Read the model definition and answer for the solid it produces. Units are mm, in the model's axes. A direction names the side the tool comes from. Coordinates: 2 decimals unless noted, no trailing zeros. Loops run counter-clockwise (first coordinate to the right, second up) from the corner with the lowest first, then second, coordinate; pieces in that order, holes last. Notation, with made-up numbers: M 59,69.25 L 72,69.25 A21 cw 72,76.25 Z; hole C -11.75,55.25 d10. An arc over 180 degrees is marked long. Put each result on its own line as item: value.
from build123d import *

# Parameters (mm, degrees)
F0_W     = 76.2
F0_H     = 38.1
F1_DEPTH = 2.032
F2_R     = 3.81
F3_DEPTH = 25.4
F2_W     = 71.628
F2_H     = 33.528
F2_W_2   = 67.564
F2_H_2   = 29.464
F4_DEPTH = 2.54
F5_R     = 5.08
F7_DEPTH = 25.4
F8_DEPTH = 25.4


with BuildPart() as f1:
    # F0 (on Top) → F1 (new body)
    with BuildSketch(Plane.XY):
        Rectangle(F0_W, F0_H)
    extrude(amount=F1_DEPTH)

    # F2 (on face) → F3 (cut)
    with BuildSketch(Plane.XY.offset(2.032)):
        Circle(F2_R)
    extrude(amount=-F3_DEPTH, mode=Mode.SUBTRACT)

    # F2 (on face) → F4 (join)
    with BuildSketch(Plane.XY.offset(2.032)):
        Rectangle(F2_W, F2_H)
        Rectangle(F2_W_2, F2_H_2, mode=Mode.SUBTRACT)
    extrude(amount=F4_DEPTH)

    # F5
    f5_edges = [f1.edges().sort_by_distance(p)[0] for p in [
        (-33.782, 14.732, 3.302),
        (-33.782, -14.732, 3.302),
        (33.782, -14.732, 3.302),
        (33.782, 14.732, 3.302),
        (-35.814, -16.764, 3.302),
        (-38.1, -19.05, 1.016),
        (38.1, -19.05, 1.016),
        (35.814, -16.764, 3.302),
        (38.1, 19.05, 1.016),
        (35.814, 16.764, 3.302),
        (-35.814, 16.764, 3.302),
        (-38.1, 19.05, 1.016),
    ]]
    fillet(f5_edges, radius=F5_R)

    # F6 (on face) → F7 (cut)
    with BuildSketch(Plane.XY.offset(2.032)):
        with BuildLine():
            ThreePointArc((22.9948570038, 2.5340882153), (21.082, 3.175), (19.1691429962, 2.5340882153))
            ThreePointArc((19.1691429962, 2.5340882153), (21.082, 2.1601883081), (22.9948570038, 2.5340882153))
        make_face()
        with BuildLine():
            ThreePointArc((19.1691429962, 2.5340882153), (18.2399984177, 1.4155041527), (17.907, 0))
            ThreePointArc((17.907, 0), (21.082, -3.175), (24.257, 0))
            ThreePointArc((24.257, 0), (23.9240015823, 1.4155041527), (22.9948570038, 2.5340882153))
            ThreePointArc((22.9948570038, 2.5340882153), (21.082, 2.1601883081), (19.1691429962, 2.5340882153))
        make_face()
        with BuildLine():
            ThreePointArc((17.907, 3.2746145791), (18.511267216, 2.8586665458), (19.1691429962, 2.5340882153))
            ThreePointArc((19.1691429962, 2.5340882153), (21.082, 3.175), (22.9948570038, 2.5340882153))
            ThreePointArc((22.9948570038, 2.5340882153), (23.652732784, 2.8586665458), (24.257, 3.2746145791))
            ThreePointArc((24.257, 3.2746145791), (25.6610501198, 5.0404837824), (26.162, 7.2401883081))
            ThreePointArc((26.162, 7.2401883081), (18.8822954744, 11.8192384279), (17.907, 3.2746145791))
        make_face()
        with BuildLine():
            Line((17.907, 3.2746145791), (17.907, 0))
            ThreePointArc((17.907, 0), (18.2399984177, 1.4155041527), (19.1691429962, 2.5340882153))
            ThreePointArc((19.1691429962, 2.5340882153), (18.511267216, 2.8586665458), (17.907, 3.2746145791))
        make_face()
        with BuildLine():
            ThreePointArc((22.9948570038, 2.5340882153), (23.9240015823, 1.4155041527), (24.257, 0))
            Line((24.257, 0), (24.257, 3.2746145791))
            ThreePointArc((24.257, 3.2746145791), (23.652732784, 2.8586665458), (22.9948570038, 2.5340882153))
        make_face()
    extrude(amount=-F7_DEPTH, mode=Mode.SUBTRACT)

    # F6 (on face) → F8 (cut)
    with BuildSketch(Plane.XY.offset(2.032)):
        with BuildLine():
            ThreePointArc((-24.257, 3.2746145791), (-23.652732784, 2.8586665458), (-22.9948570038, 2.5340882153))
            ThreePointArc((-22.9948570038, 2.5340882153), (-21.082, 3.175), (-19.1691429962, 2.5340882153))
            ThreePointArc((-19.1691429962, 2.5340882153), (-18.511267216, 2.8586665458), (-17.907, 3.2746145791))
            ThreePointArc((-17.907, 3.2746145791), (-16.5029498802, 5.0404837824), (-16.002, 7.2401883081))
            ThreePointArc((-16.002, 7.2401883081), (-23.2817045256, 11.8192384279), (-24.257, 3.2746145791))
        make_face()
        with BuildLine():
            ThreePointArc((-22.9948570038, 2.5340882153), (-23.9240015823, 1.4155041527), (-24.257, 0))
            ThreePointArc((-24.257, 0), (-21.082, -3.175), (-17.907, 0))
            ThreePointArc((-17.907, 0), (-18.2399984177, 1.4155041527), (-19.1691429962, 2.5340882153))
            ThreePointArc((-19.1691429962, 2.5340882153), (-21.082, 2.1601883081), (-22.9948570038, 2.5340882153))
        make_face()
        with BuildLine():
            Line((-24.257, 3.2746145791), (-24.257, 0))
            ThreePointArc((-24.257, 0), (-23.9240015823, 1.4155041527), (-22.9948570038, 2.5340882153))
            ThreePointArc((-22.9948570038, 2.5340882153), (-23.652732784, 2.8586665458), (-24.257, 3.2746145791))
        make_face()
        with BuildLine():
            ThreePointArc((-19.1691429962, 2.5340882153), (-21.082, 3.175), (-22.9948570038, 2.5340882153))
            ThreePointArc((-22.9948570038, 2.5340882153), (-21.082, 2.1601883081), (-19.1691429962, 2.5340882153))
        make_face()
        with BuildLine():
            ThreePointArc((-19.1691429962, 2.5340882153), (-18.2399984177, 1.4155041527), (-17.907, 0))
            Line((-17.907, 0), (-17.907, 3.2746145791))
            ThreePointArc((-17.907, 3.2746145791), (-18.511267216, 2.8586665458), (-19.1691429962, 2.5340882153))
        make_face()
    extrude(amount=-F8_DEPTH, mode=Mode.SUBTRACT)


solid = f1.part
1) Given pin 1 Ø0.8 at (y, z) = (0.5, 3.5) entering from -X; pin 2 Ø6 at (x, y) = (0, 0) entering from +Z; pin 3 Ø1.3 at (x, z) = (-5, 3.5) entering from -Y; pin 4 Ø0.8 at (y, z) = (2, 3.5) entering from +X, each flat-ended and moving along its own axis, determine where each tip first touches the part or whether it passes through.
Answer list:
pin 1: stops at x = -35.81
pin 2: passes through
pin 3: stops at y = -16.76
pin 4: stops at x = 35.81
2) Find section C-C, the plane y = -7.5. Write down the section's boundary in (x, z).
Answer list:
outline: M -38.1,0 L 38.1,0 L 38.1,2.03 L 35.81,2.03 L 35.81,4.57 L 33.78,4.57 L 33.78,2.03 L -33.78,2.03 L -33.78,4.57 L -35.81,4.57 L -35.81,2.03 L -38.1,2.03 Z
3) Which of the six approach directions +Z, -Z, +X, -X, +Y, -Y give full straight-line access (tool end or side, diameter ignored) to faces 5 (the cylindrical face through (21.012, -3.174, 1.03)), 6 (the cylindrical face through (32.333, -13.204, 3.32)), 7 (the flat face through (-35.814, 0, 3)), 8 (the cylindrical face through (34.3, -15.3, 3.3))?
Answer list:
face 5: +Z, -Z
face 6: +Z
face 7: +Z, -X, +Y, -Y
face 8: +Z, +X, -Y
4) Find section D-D, the plane x = -14.5. Write down the section's boundary in (y, z), plus the area to 3 significant figures.
Answer list:
outline: M -19.05,0 L 19.05,0 L 19.05,2.03 L 16.76,2.03 L 16.76,4.57 L 14.73,4.57 L 14.73,2.03 L -14.73,2.03 L -14.73,4.57 L -16.76,4.57 L -16.76,2.03 L -19.05,2.03 Z
area: 87.7 mm^2
5) Determine the mould class of faces 1 (the flat face through (-17.907, 2, 1)), 2 (the cylindrical face through (-36.651, -17.522, 1.03)), 3 (the cylindrical face through (32.254, 13.283, 3.32)), 4 (the flat face through (0, 19.05, 1)) for opening direction X: released by +X, released by -X, zero draft, split by the parting line, or undercut.
Answer list:
face 1: undercut
face 2: released by -X
face 3: undercut
face 4: zero draft
6) Find section A-A, the plane x = 0. Write down the section's boundary in (y, z).
Answer list:
outline: M -19.05,0 L -3.81,0 L -3.81,2.03 L -14.73,2.03 L -14.73,4.57 L -16.76,4.57 L -16.76,2.03 L -19.05,2.03 Z; M 3.81,0 L 19.05,0 L 19.05,2.03 L 16.76,2.03 L 16.76,4.57 L 14.73,4.57 L 14.73,2.03 L 3.81,2.03 Z
7) Straight lines are drawn through the part: line 1 (X direction, y = -5, z = 3.95); line 2 (Y direction, x = 0, z = 0.9); line 3 (X direction, y = -2.5, z = 0.9). For each, find the intervals that lie inside material, in ascending order. Write a range as [from, to].
Answer list:
line 1: x = [-35.81, -33.78], [33.78, 35.81]
line 2: y = [-19.05, -3.81], [3.81, 19.05]
line 3: x = [-38.1, -23.04], [-19.12, -2.88], [2.88, 19.12], [23.04, 38.1]
8) Find section B-B, the plane z = 1.25. Write down the section's boundary in (x, y) (3 decimals).
Answer list:
outline: M -38.1,-13.97 A5.08 ccw -33.02,-19.05 L 33.02,-19.05 A5.08 ccw 38.1,-13.97 L 38.1,13.97 A5.08 ccw 33.02,19.05 L -33.02,19.05 A5.08 ccw -38.1,13.97 Z; hole M -24.257,0 A3.175 ccw -17.907,0 L -17.907,3.275 A5.08 ccw long -24.257,3.275 Z; hole C 0,0 d7.62; hole M 17.907,0 A3.175 ccw 24.257,0 L 24.257,3.275 A5.08 ccw long 17.907,3.275 Z
